Verification items for the finished model (mm, model axes). A direction names the side the tool comes from. Round coordinates to 2 decimals unless told otherwise and drop trailing zeros. Write each loop counter-clockwise with the first axis right and the second up, starting at its lowest first coordinate (ties: lowest second). Pieces come first, ordered by that corner, then holes. Notation, with made-up numbers: (61.25, 14.25) -> (108.25, 14.25) arc R26 ccw to (108.25, 29.25) -> close; hole circle Ø7 at (-7, 29). An arc over 180 degrees is marked (long way). Use CSV: the item, a comma, the result in double quotes.
```python
from build123d import *

# Parameters (mm, degrees)
SKETCH1_R            = 8.89
SKETCH1_R_2          = 6.35
BOSS_EXTRUDE1_DEPTH  = 5.08
FILLET1_R            = 0.635
SKETCH2_W            = 8.89
SKETCH2_H            = 3.81
BOSS_EXTRUDE2_DEPTH  = 3.81
BOSS_EXTRUDE3_START  = -3.175
SKETCH3_W            = 2.54
SKETCH3_H            = 8.89
BOSS_EXTRUDE3_DEPTH  = 13.335
FILLET2_R            = 4.445
SKETCH4_R            = 3.175
CUT_EXTRUDE1_DEPTH   = 10.16
FILLET2_OF_MIRROR1_R = 4.445


with BuildPart() as part:
    # Sketch1 → Boss-Extrude1 (new, symmetric)
    with BuildSketch(Plane.XY):
        Circle(SKETCH1_R)
        Circle(SKETCH1_R_2, mode=Mode.SUBTRACT)
    extrude(amount=BOSS_EXTRUDE1_DEPTH, both=True)

    # Fillet1
    fillet1_edges = [part.edges().sort_by_distance(p)[0] for p in [
        (-8.89, 0, -5.08),
        (-8.89, 0, 5.08),
    ]]
    fillet(fillet1_edges, radius=FILLET1_R)

    # Sketch2 → Boss-Extrude2 (add, symmetric)
    with BuildSketch(Plane(origin=(0, 0, 0), x_dir=(0, 0, -1), z_dir=(1, 0, 0))):
        with Locations((0, 8.255)):
            Rectangle(SKETCH2_W, SKETCH2_H)
    boss_extrude2 = extrude(amount=BOSS_EXTRUDE2_DEPTH, both=True)

    # Sketch3 → Boss-Extrude3 (add)
    with BuildSketch(Plane(origin=(0, 10.16, 0), x_dir=(1, 0, 0), z_dir=(0, 1, 0)).offset(BOSS_EXTRUDE3_START)):
        with Locations((3.81, 0)):
            Rectangle(SKETCH3_W, SKETCH3_H)
        with Locations((-3.81, 0)):
            Rectangle(SKETCH3_W, SKETCH3_H)
    boss_extrude3 = extrude(amount=BOSS_EXTRUDE3_DEPTH)

    # Fillet2
    fillet2_edges = [part.edges().sort_by_distance(p)[0] for p in [
        (-3.81, 20.32, -4.445),
        (-3.81, 20.32, 4.445),
        (3.81, 20.32, -4.445),
        (3.81, 20.32, 4.445),
    ]]
    fillet(fillet2_edges, radius=FILLET2_R - 0.0001)  # a hair under: the kernel refuses the full size

    # Sketch4 → Cut-Extrude1 (cut)
    with BuildSketch(Plane(origin=(5.08, 0, 0), x_dir=(0, 0, -1), z_dir=(1, 0, 0))):
        with Locations((0, 15.875)):
            Circle(SKETCH4_R)
    cut_extrude1 = extrude(amount=-CUT_EXTRUDE1_DEPTH, mode=Mode.SUBTRACT)

    # Mirror1: Boss-Extrude2, Boss-Extrude3, Cut-Extrude1 across plane
    add(boss_extrude2.mirror(Plane.ZX))
    add(boss_extrude3.mirror(Plane.ZX))
    add(cut_extrude1.mirror(Plane.ZX), mode=Mode.SUBTRACT)

    # Fillet2 of Mirror1
    fillet2_of_mirror1_edges = [part.edges().sort_by_distance(p)[0] for p in [
        (-3.81, -20.32, -4.445),
        (-3.81, -20.32, 4.445),
        (3.81, -20.32, -4.445),
        (3.81, -20.32, 4.445),
    ]]
    fillet(fillet2_of_mirror1_edges, radius=FILLET2_OF_MIRROR1_R - 0.0001)  # a hair under: the kernel refuses the full size


solid = part.part
```
Q1. Section check B-B (z = -2.5). State how many separate pieces and enclosed holes the cut face has, plus the area to 3 significant figures.
Filled in:
separate pieces,"5"
enclosed holes,"1"
area,"213 mm²"
Q2. Mould release check, pull along Y, two halves, no side actions. Record for faces 5 (the cylindrical face through (-3.79, 18.98, 3.18)), 6 (the cylindrical face through (-3.792, -19.023, 0.413)), 7 (the flat face through (2.4, -6.1, 5.08)): released by +Y, released by -Y, zero draft, split by the parting line, or undercut.
Filled in:
face 5,"released by +Y"
face 6,"undercut"
face 7,"zero draft"
Q3. Go/stop test with flat-tipped pins: P1, Ø1.5, axis at x = -1, z = -2, coming from the +Y side; P2, Ø6, axis at x = 5.5, z = 3.5, coming from the -Y side; P3, Ø4.5, axis at y = 15.5, z = -1, coming from the -X side. Record where each tip stops, or that it passes through.
Filled in:
P1,"y = 10.16"
P2,"y = -20.29"
P3,"x = -5.08"
Q4. Access from +Z, -Z, +X, -X, +Y, -Y to the whole of each face (thin tool, end or side, straight path). Record for faces 1 (the flat face through (2.54, -13, 2)), 2 (the flat face through (-5.08, 12, 0)), 3 (the flat face through (5.08, -12, 0)), 4 (the flat face through (-5.08, -12, 0)).
Filled in:
face 1,"+Z, -Z, -Y"
face 2,"+Z, -Z, -X, +Y"
face 3,"+Z, -Z, +X, -Y"
face 4,"+Z, -Z, -X, -Y"
Q5. Material ranges on L1, parallel to Y at x = 3.8, z = 0; L2, parallel to Y at x = 3, z = 1.25; L3, parallel to Y at x = -0.25, z = -1.75, recorded low to high.
Filled in:
L1,"-20.32 to -19.05, -12.7 to -5.09, 5.09 to 12.7, 19.05 to 20.32"
L2,"-20.14 to -18.79, -12.96 to -5.6, 5.6 to 12.96, 18.79 to 20.14"
L3,"-10.16 to -6.35, 6.35 to 10.16"
Q6. Section check A-A (y = 0). Record the cut outline in (x, z) (3 decimals).
Filled in:
outline,"(-8.89, -4.445) arc R0.635 ccw to (-8.255, -5.08) -> (-6.35, -5.08) -> (-6.35, 5.08) -> (-8.255, 5.08) arc R0.635 ccw to (-8.89, 4.445) -> close; (6.35, -5.08) -> (8.255, -5.08) arc R0.635 ccw to (8.89, -4.445) -> (8.89, 4.445) arc R0.635 ccw to (8.255, 5.08) -> (6.35, 5.08) -> close"
